Here's how the part is built. I have some questions about the finished solid (model axes, mm). Face numbers are marked on the shaded views. Give positions to 0.01 mm unless a question says otherwise; leave off trailing zeros. Write each loop counter-clockwise with the first axis right and the second up, starting at its lowest first coordinate (ties: lowest second). Pieces come first, ordered by that corner, then holes. Notation, with made-up numbers: (40, 21) - (86, 21) arc R21 ccw to (86, 33) - close; hole circle Ø10 at (56.5, 79). An arc over 180 degrees is marked (long way). Use a Markdown table: item, result.
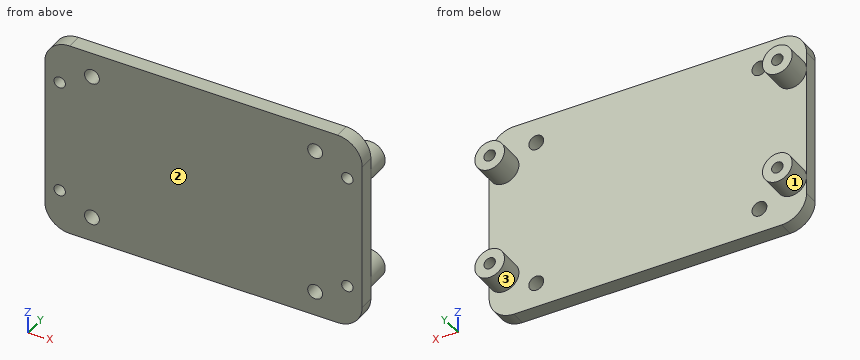
Autodesk Inventor part; units mm, degrees
ref_plane "YZ Plane" through (0, 0, 0) normal (1, 0, 0) x (0, 1, 0)
ref_plane "XZ Plane" through (0, 0, 0) normal (0, 1, 0) x (-1, 0, 0)
ref_plane "XY Plane" through (0, 0, 0) normal (0, 0, 1) x (1, 0, 0)
sketch "Sketch1" plane through (0, 0, 0) normal (0, 1, 0) x (-1, 0, 0)
  line L0 (0, 0) -> (58, 0)
  line L1 (58, 0) -> (58, -23)
  line L2 (58, -23) -> (0, -23)
  line L3 (0, -23) -> (0, 0)
  line L4 (6.5, 3.5) -> (51.5, 3.5)
  line L5 (51.5, 3.5) -> (51.5, -26.5)
  line L6 (51.5, -26.5) -> (6.5, -26.5)
  line L7 (6.5, -26.5) -> (6.5, 3.5)
  circle A0 centre (51.5, 3.5) radius 1.5
  circle A1 centre (51.5, -26.5) radius 1.5
  circle A2 centre (6.5, -26.5) radius 1.5
  circle A3 centre (6.5, 3.5) radius 1.5
  line L8 (-3, 8.5) -> (61, 8.5)
  line L9 (61, 8.5) -> (61, -31.5)
  line L10 (61, -31.5) -> (-3, -31.5)
  line L11 (-3, -31.5) -> (-3, 8.5)
  circle A4 centre (58, 0) radius 1.15
  circle A5 centre (58, -23) radius 1.15
  circle A6 centre (0, 0) radius 1.15
  circle A7 centre (0, -23) radius 1.15
  circle A8 centre (58, 0) radius 3
  circle A9 centre (58, -23) radius 3
  circle A10 centre (0, 0) radius 3
  circle A11 centre (0, -23) radius 3
  dimension "d0" = 23
  dimension "d1" = 58
  dimension "d2" = 45
  dimension "d3" = 30
  dimension "d4" = 3.5
  dimension "d6" = 3
  dimension "d7" = 3
  dimension "d8" = 3
  dimension "d9" = 3
  dimension "d10" = 9.5
  dimension "d11" = 5
  dimension "d12" = 5
  dimension "d13" = 9.5
  dimension "d14" = 2.3
  dimension "d15" = 2.3
  dimension "d16" = 2.3
  dimension "d17" = 2.3
  dimension "d18" = 6
  dimension "d19" = 6
  dimension "d20" = 6
  dimension "d21" = 6
  dimension "d28" = 6.5
extrude "Extrusion1" add sketch "Sketch1" along normal blind 3 contours A6 L3 A10 L0 | L0 A10 L3 A6 | A10 L11 L8 L9 A8 L0 L5 A0 L4 A3 L7 | L0 L7 L2 A11 L3 A10 | L3 A11 L11 A10 | L7 A3 L4 A0 L5 L0 | L0 L5 L2 L7 | A11 L2 A7 L3 | L3 A7 L2 A11 | L0 A8 L1 A9 L2 L5 | L7 A2 L6 A1 L5 L2 A9 L9 L10 L11 A11 | L2 L5 A1 L6 A2 L7 | A8 L1 A4 L0 | L0 A4 L1 A8 | L9 A9 L1 A8 | A9 L1 A5 L2 | L2 A5 L1 A9
extrude "Extrusion2" add sketch "Sketch1" along normal blind 8 contours A6 L3 A10 L0 | L0 A10 L3 A6 | A11 L2 A7 L3 | L3 A7 L2 A11 | A8 L1 A4 L0 | L0 A4 L1 A8 | A9 L1 A5 L2 | L2 A5 L1 A9
fillet "Fillet1" radius 5 4 edges at (-61, 1.5, 8.5) (3, 1.5, 8.5) (3, 1.5, -31.5) (-61, 1.5, -31.5)
properties part number "RaspberryMount"
Item 1: Thinking about a two-plate mould opening in X: for the marked faces 1, 2 and 3, which applies, +X half, -X half, draft (parallel to the pull), parting line (faces both ways), or undercut?
Values:
| item | result |
|---|---|
| face 1 | undercut |
| face 2 | draft |
| face 3 | undercut |
Item 2: If we section it at D-D, the plane z = -17.5: Write out the boundary of the cut face in (x, y).
Values:
| item | result |
|---|---|
| outline | (-61, 0) - (3, 0) - (3, 3) - (-61, 3) - close |
Item 3: If we section it at C-C, the plane x = -58: Write out the boundary of the cut face in (y, z), plus the area to 3 significant figures.
Values:
| item | result |
|---|---|
| outline | (0, -31.08) - (3, -31.08) - (3, -26) - (8, -26) - (8, -24.15) - (0, -24.15) - close; (0, -21.85) - (8, -21.85) - (8, -20) - (3, -20) - (3, -3) - (8, -3) - (8, -1.15) - (0, -1.15) - close; (0, 1.15) - (8, 1.15) - (8, 3) - (3, 3) - (3, 8.08) - (0, 8.08) - close |
| area | 141 mm2 |
Item 4: If we section it at B-B, the plane x = -6.5: Write out the boundary of the cut face in (y, z), plus the area to 3 significant figures.
Values:
| item | result |
|---|---|
| outline | (0, -31.5) - (3, -31.5) - (3, -28) - (0, -28) - close; (0, -25) - (3, -25) - (3, 2) - (0, 2) - close; (0, 5) - (3, 5) - (3, 8.5) - (0, 8.5) - close |
| area | 102 mm2 |
Item 5: Will these pins go through, and if not, where does the flat tip stop? pin 1 Ø2 at (x, y) = (-3.5, 6.5) entering from -Z; pin 2 Ø5 at (x, z) = (-6.5, 3.5) entering from +Y.
Values:
| item | result |
|---|---|
| pin 1 | stops at z = -24.66 |
| pin 2 | stops at y = 3 |
Item 6: If we section it at A-A, the plane y = 5.5: Write out the boundary of the cut face in (x, z), plus the area to 3 significant figures.
Values:
| item | result |
|---|---|
| outline | circle Ø6 at (-58, -23); circle Ø6 at (-58, 0); circle Ø6 at (0, -23); circle Ø6 at (0, 0); hole circle Ø2.3 at (-58, -23); hole circle Ø2.3 at (-58, 0); hole circle Ø2.3 at (0, -23); hole circle Ø2.3 at (0, 0) |
| area | 96.5 mm2 |
Item 7: I need wall thicknesses on line 1 along X through (y, z) = (4, -23); line 2 along X through (y, z) = (1.5, -26.5); line 3 along Z through (x, y) = (-6.5, 2.15). Which ranges of each line are inside material? Lowest first, please. Write a range as [from, to].
Values:
| item | result |
|---|---|
| line 1 | x = [-61, -59.15], [-56.85, -55], [-3, -1.15], [1.15, 3] |
| line 2 | x = [-61, -53], [-50, -8], [-5, 3] |
| line 3 | z = [-31.5, -28], [-25, 2], [5, 8.5] |
